Could you check a few things on this drawing? It's one solid part, dimensions in mm from its lowest x, y, z. Give positions to 0.01 mm unless a question says otherwise; leave off trailing zeros. Loops run counter-clockwise (first coordinate to the right, second up) from the corner with the lowest first, then second, coordinate; pieces in that order, holes last. Notation, with made-up numbers: (-29.5, 71) - (14.5, 71) arc R30 cw to (14.5, 103) - close; hole circle Ø10 at (15, -4.5). An arc over 180 degrees is marked (long way). Put each result on its own line as item: value. Start each with the question number.
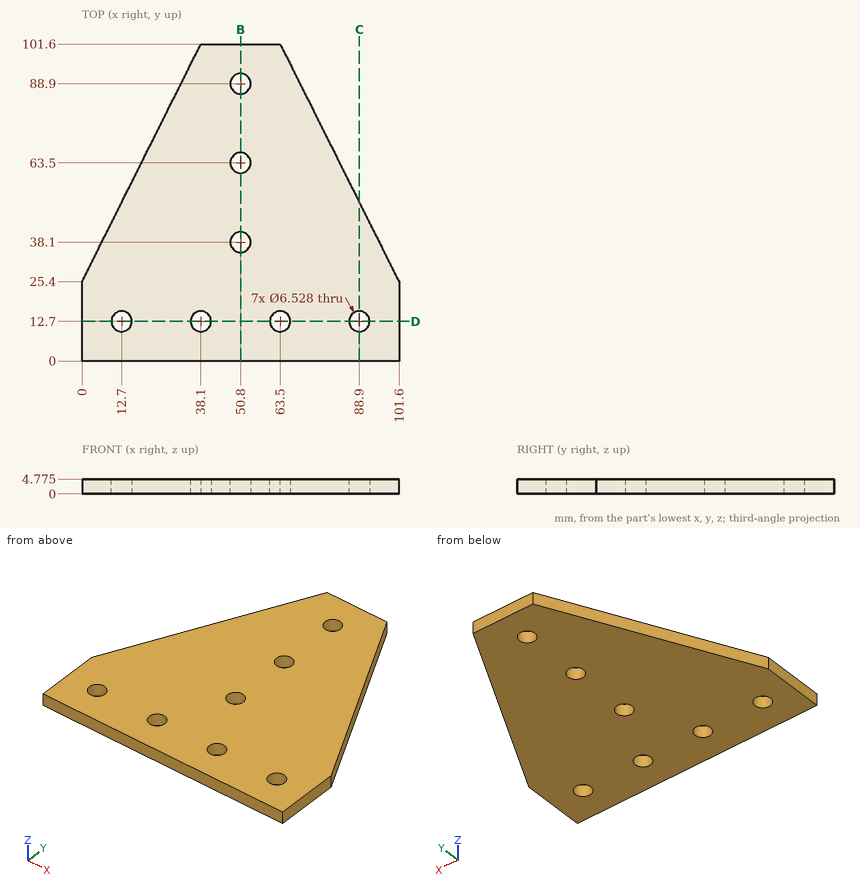
1) I need wall thicknesses on line 1 (Y direction, x = 50.8, z = 3.4); line 2 (Y direction, x = 63.5, z = 2.15) (1 decimal); line 3 (X direction, y = 11, z = 1.7). Which ranges of each line are inside material? Lowest first, please.
2) I'm going to push a flat-ended pin straight in: P1, Ø10.5, axis at x = 50.8, y = 88.9, coming from the +Z side (3 decimals). Where does the tip first touch, or does it pass through?
3) Suppose I cut it at D-D on y = 12.7. Please give me the cut outline in (x, z) (1 decimal).
4) Suppose I cut it at B-B on x = 50.8. Please give me the cut outline in (y, z) (1 decimal), plus the area to 3 significant figures.
5) Suppose I cut it at C-C on x = 88.9. Please give me the cut outline in (y, z) (1 decimal), plus the area to 3 significant figures.
Ans:
1. line 1: y = 0 to 34.84, 41.36 to 60.24, 66.76 to 85.64, 92.16 to 101.6
1. line 2: y = 0 to 9.4, 16 to 101.6
1. line 3: x = 0 to 9.91, 15.49 to 35.31, 40.89 to 60.71, 66.29 to 86.11, 91.69 to 101.6
2. P1: stops at z = 4.775
3. outline: (0, 0) - (9.4, 0) - (9.4, 4.8) - (0, 4.8) - close; (16, 0) - (34.8, 0) - (34.8, 4.8) - (16, 4.8) - close; (41.4, 0) - (60.2, 0) - (60.2, 4.8) - (41.4, 4.8) - close; (66.8, 0) - (85.6, 0) - (85.6, 4.8) - (66.8, 4.8) - close; (92.2, 0) - (101.6, 0) - (101.6, 4.8) - (92.2, 4.8) - close
4. outline: (0, 0) - (34.8, 0) - (34.8, 4.8) - (0, 4.8) - close; (41.4, 0) - (60.2, 0) - (60.2, 4.8) - (41.4, 4.8) - close; (66.8, 0) - (85.6, 0) - (85.6, 4.8) - (66.8, 4.8) - close; (92.2, 0) - (101.6, 0) - (101.6, 4.8) - (92.2, 4.8) - close
4. area: 392 mm²
5. outline: (0, 0) - (9.4, 0) - (9.4, 4.8) - (0, 4.8) - close; (16, 0) - (50.8, 0) - (50.8, 4.8) - (16, 4.8) - close
5. area: 211 mm²
